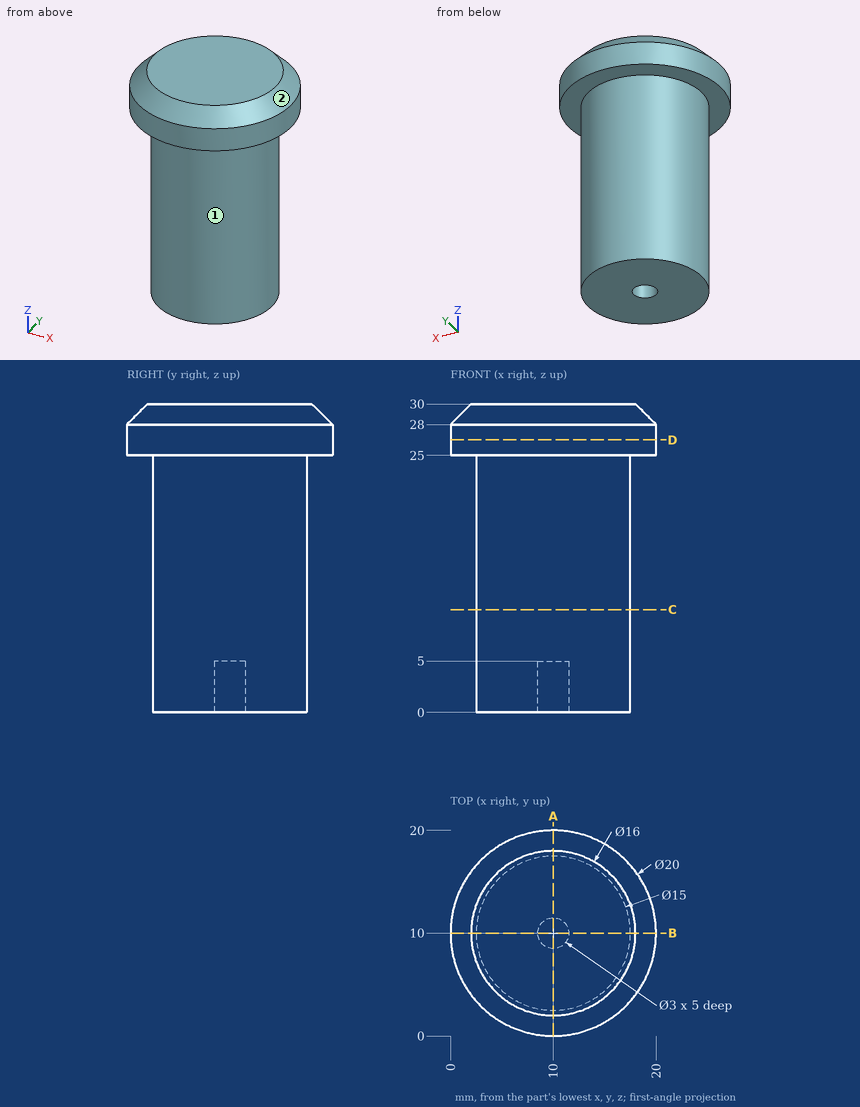
Study the drawing (mm; zero at the part's minimum x, y, z) and answer. A direction names the side the tool comes from. Coordinates: 2 decimals unless noted, no trailing zeros. Write each loop counter-clockwise with the first axis right and the second up, starting at its lowest first coordinate (ties: lowest second). Pieces come first, ordered by that corner, then holes. Notation, with made-up numbers: (48.5, 5) - (53.5, 5) arc R16 ccw to (53.5, 33) - close; hole circle Ø10 at (20, 67.5). An arc over 180 degrees is marked (long way). One line per item, written item: value.
1) Consider line 1 along Y through (x, z) = (10, 1.3); line 2 along Y through (x, z) = (9.75, 20.5); line 3 along Z through (x, y) = (2, 14). Determine where each line is inside the solid, lowest interval first. Write a range as from..to.
Geometry check:
line 1: y = 2.5..8.5, 11.5..17.5
line 2: y = 2.5..17.5
line 3: z = 25..29.06
2) Find section A-A (x = 10). Give the vertices of the cut face in (y, z), and give its area (3 significant figures).
Geometry check:
outline: (0, 25) - (2.5, 25) - (2.5, 0) - (8.5, 0) - (8.5, 5) - (11.5, 5) - (11.5, 0) - (17.5, 0) - (17.5, 25) - (20, 25) - (20, 28) - (18, 30) - (2, 30) - (0, 28) - close
area: 456 mm2
3) Find section D-D (z = 26.5). Give the vertices of the cut face in (x, y).
Geometry check:
outline: circle Ø20 at (10, 10)
4) A tool of negligible diameter and unlimited length cuts with its end or side. For the marked faces 1 and 2, from which of +Z, -Z, +X, -X, +Y, -Y can it reach the whole face along a straight path? Write none if from no direction.
Geometry check:
face 1: -Z
face 2: +Z
5) Find section C-C (z = 10). Give the vertices of the cut face in (x, y), and give its area (3 significant figures).
Geometry check:
outline: circle Ø15 at (10, 10)
area: 177 mm2
6) Each of these flat-tipped pins is pushed along its axis until it touches: pin 1 Ø1 at (y, z) = (13.5, 8.5) entering from -X; pin 2 Ø4 at (y, z) = (16.5, 16) entering from +X; pin 3 Ø5 at (x, z) = (6, 16) entering from -Y. Where does it stop, or does it pass through?
Geometry check:
pin 1: stops at x = 3.13
pin 2: stops at x = 16
pin 3: stops at y = 2.65
